Input: part model. Units: mm. Frame: model coordinates. Round coordinates to 2 decimals unless told otherwise and drop trailing zeros. Loops run counter-clockwise (first coordinate to the right, second up) from the corner with the lowest first, then second, coordinate; pieces in that order, holes last.
1) Section A-A, the plane x = 13.25. Return loops of the section in (y, z).
2) Section C-C, the plane y = 303. Return loops of the section in (x, z), and give its area (3 significant figures).
3) Ray query, line 1 along X through (y, z) = (323, 16.5). Return the intervals inside material, ascending.
4) Section B-B, the plane z = 11.5. Return loops of the section in (x, y).
Autodesk Inventor part; units mm, degrees
ref_plane "YZ Plane" through (0, 0, 0) normal (1, 0, 0) x (0, 1, 0)
ref_plane "XZ Plane" through (0, 0, 0) normal (0, 1, 0) x (-1, 0, 0)
ref_plane "XY Plane" through (0, 0, 0) normal (0, 0, 1) x (1, 0, 0)
sketch "Sketch1" plane through (0, 0, 0) normal (0, 0, 1) x (1, 0, 0)
  line L0 (0, 0) -> (19, 0)
  line L1 (19, 0) -> (19, 400)
  line L2 (19, 400) -> (0, 400)
  line L3 (0, 400) -> (0, 0)
  dimension "d0" = 19
  dimension "d1" = 400
extrude "Extrusion1" add sketch "Sketch1" along normal blind 19
sketch "Sketch2" plane through (0, 400, 0) normal (0, 1, 0) x (1, 0, 0)
  line L0 (19, 0) -> (0, 0)
  line L1 (0, 0) -> (0, -19)
  line L2 (19, -19) -> (0, -19)
  line L3 (19, 0) -> (19, -19)
  line L4 (1.5, -17.5) -> (1.5, -1.5)
  line L5 (1.5, -1.5) -> (17.5, -1.5)
  line L6 (17.5, -1.5) -> (17.5, -17.5)
  line L7 (17.5, -17.5) -> (1.5, -17.5)
  point P0 (0, 0)
  dimension "d4" = 1.5
extrude "Extrusion2" cut sketch "Sketch2" against normal through all contours L4 L5 L6 L7
properties part number "C001" material "Aluminum 6061"
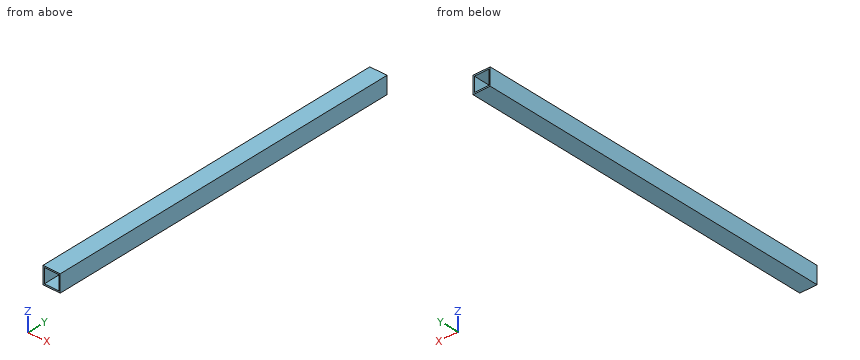
Final values:
1. outline: (0, 0) - (400, 0) - (400, 1.5) - (0, 1.5) - close; (0, 17.5) - (400, 17.5) - (400, 19) - (0, 19) - close
2. outline: (0, 0) - (19, 0) - (19, 19) - (0, 19) - close; hole (1.5, 1.5) - (17.5, 1.5) - (17.5, 17.5) - (1.5, 17.5) - close
2. area: 105 mm2
3. line 1: x = 0 to 1.5, 17.5 to 19
4. outline: (0, 0) - (1.5, 0) - (1.5, 400) - (0, 400) - close; (17.5, 0) - (19, 0) - (19, 400) - (17.5, 400) - close
